Model file for the job. Use its own axes, mm. A direction names the side the tool comes from. Round coordinates to 2 decimals unless told otherwise and drop trailing zeros. Loops run counter-clockwise (first coordinate to the right, second up) from the corner with the lowest first, then second, coordinate; pieces in that order, holes last. Notation, with made-up numbers: M 69.5,4 L 109.5,4 A29 cw 109.5,26 Z; hole C -23.5,74 d4. An arc over 180 degrees is marked long. Answer in a Markdown table with one row per item.
Autodesk Fusion 360 part; units mm, degrees
sketch "Sketch1" plane through (0, 0, 0) normal (0, 0, 1) x (1, 0, 0)
  line L0 (0, 0) -> (17, 0)
  line L1 (17, 0) -> (17, 200)
  line L2 (17, 200) -> (0, 200)
  line L3 (0, 200) -> (0, 0)
  line L4 (5, 0) -> (5, 200)
  line L5 (12, 0) -> (12, 200)
  dimension "d1" = 17
  dimension "d2" = 200
  dimension "d3" = 200
  dimension "d4" = 7
  dimension "d5" = 200
extrude "Extrude1" add sketch "Sketch1" along normal blind 5
sketch "Sketch2" plane through (0, 0, 5) normal (0, 0, 1) x (-1, 0, 0)
  line L0 (0, -200) -> (0, 0)
  line L1 (0, 0) -> (-17, 0)
  line L2 (-17, 0) -> (-17, -200)
  line L3 (-17, -200) -> (0, -200)
  line L4 (-5, 0) -> (-5, -200)
  line L5 (-12, 0) -> (-12, -200)
  dimension "d8" = 5
  dimension "d9" = 7
  dimension "d10" = 200
  dimension "d11" = 200
extrude "Extrude2" add sketch "Sketch2" along normal blind 12 contours L0 L1 L3 L4 | L1 L2 L3 L5
sketch "Sketch3" plane through (12, 0, 0) normal (-1, 0, 0) x (0, -1, 0)
  line L0 (-200, 5) -> (0, 5)
  line L1 (0, 5) -> (0, 17)
  line L2 (0, 17) -> (-200, 17)
  line L3 (-200, 17) -> (-200, 5)
  line L4 (0, 17) -> (0, 12)
  line L5 (0, 12) -> (-200, 12)
  dimension "d14" = 200
extrude "Extrude3" add sketch "Sketch3" along normal blind 7 contours L1 L2 L3 L4 L5
move_face "OffsetFaces1" offset -0.5 4 faces at (12, 133.3333, 9.6667) (9.6667, 66.6667, 12) (5, 133.3333, 9.6667) (7.3333, 133.3333, 5)
sketch "Sketch4" plane through (0, 0, 17) normal (0, 0, 1) x (-1, 0, 0)
  line L0 (-17, -200) -> (0, -200)
  line L1 (0, -200) -> (0, 0)
  line L2 (0, 0) -> (-17, 0)
  line L3 (-17, 0) -> (-17, -200)
  line L4 (25, 0) -> (25, -200)
  line L5 (-42, 0) -> (-42, -200)
  line L6 (25, -200) -> (-42, -200)
  line L7 (25, 0) -> (-42, 0)
  dimension "d18" = 25
  dimension "d19" = 25
extrude "Extrude4" add sketch "Sketch4" along normal blind 2.5
move_face "OffsetFaces2" offset -3 3 faces at (17, 133.3333, 11.3333) (5.6667, 133.3333, 0) (0, 133.3333, 5.6667)
move_face "MoveFace1" by (0, 0, 3) 4 faces at (9.8333, 66.6667, 12.5) (4.5, 133.3333, 9.8333) (7.1667, 133.3333, 4.5) (12.5, 133.3333, 9.8333)
extrude "Extrude5" cut 1 faces at (6.6667, 133.3333, 3) along direction (0, 0, 1) blind 3
extrude "Extrude6" cut 1 faces at (19.6667, 133.3333, 19.5) along direction (0, 0, -1) blind 1
move_face "OffsetFaces3" offset 0.5 4 faces at (12.5, 133.3333, 12.8333) (7.1667, 133.3333, 7.5) (9.8333, 66.6667, 15.5) (4.5, 133.3333, 12.8333)
move_face "OffsetFaces4" offset 1 4 faces at (5, 133.3333, 12.6667) (7.3333, 133.3333, 8) (12, 133.3333, 12.6667) (7.3333, 66.6667, 15)
move_face "OffsetFaces5" offset -0.5 4 faces at (11, 133.3333, 12.3333) (9.3333, 66.6667, 14) (6, 133.3333, 12.3333) (7.6667, 133.3333, 9)
move_face "OffsetFaces6" offset -0.5 3 faces at (14, 66.6667, 9.6667) (6.6667, 133.3333, 6) (3, 66.6667, 13.3333)
move_face "OffsetFaces7" offset -0.5 3 faces at (13.5, 66.6667, 10) (6.8333, 133.3333, 6.5) (3.5, 66.6667, 13.5)
move_face "OffsetFaces8" offset -0.5 3 faces at (13, 66.6667, 10.3333) (7, 133.3333, 7) (4, 66.6667, 13.6667)
move_face "MoveFace2" by (0, 0, 3) 4 faces at (11.5, 133.3333, 12.5) (7.5, 66.6667, 14.5) (7.5, 133.3333, 8.5) (5.5, 133.3333, 12.5)
move_face "OffsetFaces9" offset -3 1 faces at (7.1667, 133.3333, 7.5)
move_face "OffsetFaces10" offset -0.5 2 faces at (32.1667, 133.3333, 17) (-5.3333, 66.6667, 17)
extrude "Extrude7" add 1 faces at (7.1667, 133.3333, 10.5) along direction (0, 0, -1) blind 0.5
move_face "MoveFace3" by (0, 0, -0.5) 4 faces at (11.5, 66.6667, 13.5) (7.5, 66.6667, 17.5) (5.5, 66.6667, 13.5) (7.5, 133.3333, 11.5)
move_face "OffsetFaces11" offset -4.5 1 faces at (42, 66.6667, 17.8333)
move_face "OffsetFaces12" offset -4.5 1 faces at (-25, 66.6667, 17.8333)
move_face "OffsetFaces13" offset 50 1 faces at (7.1667, 0, 18.1667)
move_face "OffsetFaces14" offset -0.5 4 faces at (11.5, 116.6667, 15) (7.5, 116.6667, 11) (5.5, 116.6667, 15) (9.5, 33.3333, 17)
move_face "OffsetFaces15" offset 0.5 3 faces at (12.5, 33.3333, 12.5) (7.1667, 116.6667, 10) (4.5, 116.6667, 15)
move_face "OffsetFaces16" offset 0.5 1 faces at (10, 33.3333, 9.5)
move_face "MoveFace4" by (0, 0, -0.5) 4 faces at (12, 33.3333, 15.1667) (9.6667, 33.3333, 10.5) (5, 33.3333, 15.1667) (7.3333, 116.6667, 17.5)
move_face "OffsetFaces17" offset 0.5 4 faces at (12, 33.3333, 14.6667) (7.3333, 116.6667, 17) (5, 33.3333, 14.6667) (9.6667, 33.3333, 10)
move_face "MoveFace5" by (0, 0, 0.5) 4 faces at (5.5, 116.6667, 14.5) (7.5, 116.6667, 10.5) (11.5, 116.6667, 14.5) (9.5, 33.3333, 16.5)
move_face "OffsetFaces18" offset -0.5 1 faces at (10, 33.3333, 9)
move_face "OffsetFaces19" offset -0.02 1 faces at (7.5, 116.6667, 11)
move_face "OffsetFaces20" offset -0.2 2 faces at (11.5, 116.6667, 14.9933) (5.5, 116.6667, 14.9933)
move_face "OffsetFaces21" offset -0.18 2 faces at (9.5667, 33.3333, 17) (7.4333, 116.6667, 10.98)
move_face "OffsetFaces22" offset 0.18 1 faces at (9.5667, 33.3333, 17.18)
move_face "OffsetFaces23" offset 0.1 2 faces at (11.7, 33.3333, 12.8667) (5.3, 33.3333, 12.8667)
move_face "OffsetFaces24" offset 0.1 2 faces at (13, 116.6667, 14.8333) (4, 33.3333, 12.1667)
move_face "OffsetFaces25" offset 0.2 1 faces at (6.9667, 116.6667, 9.5)
move_face "OffsetFaces26" offset -1 1 faces at (18.1667, 116.6667, 18.5)
move_face "OffsetFaces27" offset -202.2 1 faces at (7.4667, -50, 9.8)
move_face "OffsetFaces28" offset 1 1 faces at (7.4667, 152.2, 9.8)
move_face "OffsetFaces29" offset -0.4 4 faces at (11.6, 167.4667, 12.8667) (9.5333, 183.7333, 17) (5.4, 167.4667, 12.8667) (7.4667, 183.7333, 10.8)
1. Saw through at C-C (y = 162). Write the cut outline in (x, z).
Verdict:
| item | result |
|---|---|
| outline | M 3.9,9.3 L 13.1,9.3 L 13.1,17.5 L 3.9,17.5 Z; hole M 5,10.4 L 12,10.4 L 12,17.4 L 5,17.4 Z |
2. Saw through at B-B (z = 12.5). Write the cut outline in (x, y).
Verdict:
| item | result |
|---|---|
| outline | M 3.9,151.2 L 5,151.2 L 5,200 L 3.9,200 Z; M 12,151.2 L 13.1,151.2 L 13.1,200 L 12,200 Z |
3. Mould opens along X. For faces 3 (the flat face through (8, 176, 9.3)), 4 (the flat face through (5, 175, 14)), 5 (the flat face through (13.1, 175, 13)) say: +X half, -X half, draft (parallel to the pull), parting line (faces both ways), or undercut.
Verdict:
| item | result |
|---|---|
| face 3 | draft |
| face 4 | undercut |
| face 5 | +X half |
4. Tool access for faces 1 (the flat face through (8, 176, 10.4)), 2 (the flat face through (8, 151.2, 10)): list every direction of +Z, -Z, +X, -X, +Y, -Y with a clear straight run to the whole face (end or side of a thin tool).
Verdict:
| item | result |
|---|---|
| face 1 | +Y, -Y |
| face 2 | +Z, -Z, +X, -X, -Y |
5. Saw through at A-A (x = 7.25). Write the cut outline in (y, z), and give its area (3 significant figures).
Verdict:
| item | result |
|---|---|
| outline | M 151.2,9.3 L 200,9.3 L 200,10.4 L 151.2,10.4 Z; M 151.2,17.4 L 200,17.4 L 200,17.5 L 151.2,17.5 Z |
| area | 58.6 mm² |
6. Pin check, flat tip, straight feed: pin 1 (1.5 mm diameter, centred on x = 8.5, z = 13, fed in from -Y). Stop position of the tip, or through.
Verdict:
| item | result |
|---|---|
| pin 1 | passes through |
7. Wall check: probe 1 along X at (y, z) = (160.5, 15.75). Give the ranges that are in metal, low to high.
Verdict:
| item | result |
|---|---|
| probe 1 | x = 3.9 to 5, 12 to 13.1 |
